```python
from build123d import *

# Parameters (mm, degrees)
SKETCH_1_R               = 16
SKETCH_1_R_2             = 6.65
EXTRUDE_1_DEPTH          = 24
SKETCH_3_R               = 1.5
CUT_EXTRUDE_2_DEPTH      = 33.984845005
PATTERN_CIRCULAR_1_COUNT = 6
EXTRUDE_START            = -24
EXTRUDE_2_DEPTH          = 24
SKETCH_7_R               = 13
CUT_EXTRUDE_3_DEPTH      = 21.8
EXTRUDE_START_2          = 13.8
SKETCH_15_R              = 13
SKETCH_15_R_2            = 12.25
EXTRUDE_4_DEPTH          = 13.8
SKETCH_11_W              = 20
SKETCH_11_H              = 8.5
CUT_EXTRUDE_4_DEPTH      = 10
FILLET_1_R               = 3
SKETCH_12_R              = 1
CUT_EXTRUDE_5_DEPTH      = 44.081318457
HOLE_WIZARD_M3_1_D       = 2.5
CHAMFER_1_SIZE           = 0.5
SKETCH_19_R              = 11
EXTRUDE_8_DEPTH          = 24
SKETCH_20_R              = 11
CUT_EXTRUDE_8_DEPTH      = 47
SKETCH_21_R              = 11
CUT_EXTRUDE_9_DEPTH      = 60
SKETCH_22_R              = 9.5
CUT_EXTRUDE_10_DEPTH     = 60


with BuildPart() as part:
    # 草图1 → 凸台-拉伸1 (new body)
    with BuildSketch(Plane.XY):
        Circle(SKETCH_1_R)
        Circle(SKETCH_1_R_2, mode=Mode.SUBTRACT)
    extrude(amount=EXTRUDE_1_DEPTH)

    # 草图3 → 切除-拉伸2 (cut, through all)
    with BuildSketch(Plane(origin=(0, 0, 0), x_dir=(-1, 0, 0), z_dir=(0, 0, -1))):
        with Locations((0, 9.5)):
            Circle(SKETCH_3_R)
    cut_extrude_2 = extrude(amount=-CUT_EXTRUDE_2_DEPTH, mode=Mode.SUBTRACT)

    # 阵列(圆周)1: 切除-拉伸2 ×6 about axis
    pattern_circular_1_axis = Axis((0, 0, 0), (0, 0, 1))
    for i in range(1, PATTERN_CIRCULAR_1_COUNT):
        add(cut_extrude_2.rotate(pattern_circular_1_axis, i * 360 / PATTERN_CIRCULAR_1_COUNT), mode=Mode.SUBTRACT)

    # 草图4 → 凸台-拉伸2 (add)
    with BuildSketch(Plane.XY.offset(24).offset(EXTRUDE_START)):
        with BuildLine():
            ThreePointArc((16, 0), (11.313708518, -11.31370848), (5.5e-08, -16))
            Line((5.5e-08, -16), (16, -16))
            Line((16, -16), (16, 0))
        make_face()
        with BuildLine():
            ThreePointArc((5.5e-08, -16), (-11.31370848, -11.313708518), (-16, 0))
            Line((-16, 0), (-16, -16))
            Line((-16, -16), (5.5e-08, -16))
        make_face()
        with BuildLine():
            Line((-16, 16), (-16, 0))
            ThreePointArc((-16, 0), (-11.313708518, 11.31370848), (-5.5e-08, 16))
            Line((-5.5e-08, 16), (-16, 16))
        make_face()
        with BuildLine():
            Line((16, 16), (-5.5e-08, 16))
            ThreePointArc((-5.5e-08, 16), (11.31370848, 11.313708518), (16, 0))
            Line((16, 0), (16, 16))
        make_face()
    extrude(amount=EXTRUDE_2_DEPTH)

    # 草图7 → 切除-拉伸3 (cut)
    with BuildSketch(Plane.XY.offset(24)):
        Circle(SKETCH_7_R)
    extrude(amount=-CUT_EXTRUDE_3_DEPTH, mode=Mode.SUBTRACT)

    # 草图15 → 凸台-拉伸4 (add)
    with BuildSketch(Plane.XY.offset(2.2).offset(EXTRUDE_START_2)):
        Circle(SKETCH_15_R)
        Circle(SKETCH_15_R_2, mode=Mode.SUBTRACT)
    extrude(amount=-EXTRUDE_4_DEPTH)

    # 草图11 → 切除-拉伸4 (cut)
    with BuildSketch(Plane(origin=(0, 16, 0), x_dir=(1, 0, 0), z_dir=(0, 1, 0))):
        with Locations((0, -9.75)):
            Rectangle(SKETCH_11_W, SKETCH_11_H)
    extrude(amount=-CUT_EXTRUDE_4_DEPTH, mode=Mode.SUBTRACT)

    # 圆角1
    fillet_1_edges = [part.edges().sort_by_distance(p)[0] for p in [
        (10, 11.537742925, 5.5),
        (10, 11.537742925, 14),
        (-10, 11.537742925, 14),
        (-10, 11.537742925, 5.5),
    ]]
    fillet(fillet_1_edges, radius=FILLET_1_R)

    # 草图12 → 切除-拉伸5 (cut, through all)
    with BuildSketch(Plane(origin=(0, 16, 0), x_dir=(1, 0, 0), z_dir=(0, 1, 0))):
        with Locations(Location((8, -3.5, 0), (0, 0, 180))):
            Circle(SKETCH_12_R)
        with Locations(Location((8, -19.5, 0), (0, 0, 180))):
            Circle(SKETCH_12_R)
        with Locations(Location((-8, -3.5, 0), (0, 0, 180))):
            Circle(SKETCH_12_R)
        with Locations(Location((-8, -19.5, 0), (0, 0, 180))):
            Circle(SKETCH_12_R)
    extrude(amount=-CUT_EXTRUDE_5_DEPTH, mode=Mode.SUBTRACT)

    # M3 螺纹孔1 (through all)
    with Locations(Plane(origin=(0, 16, 0), x_dir=(1, 0, 0), z_dir=(0, 1, 0))):
        with Locations((8, -3.5), (-8, -3.5), (-8, -19.5), (8, -19.5)):
            Hole(HOLE_WIZARD_M3_1_D / 2)

    # 倒角1
    chamfer_1_edges = [part.edges().sort_by_distance(p)[0] for p in [
        (0, -16, 24),
        (16, -16, 12),
        (16, 0, 0),
        (16, 0, 24),
        (0, -16, 0),
        (-16, -16, 12),
        (-16, 0, 24),
        (-16, 0, 0),
        (0, 16, 0),
        (-16, 16, 12),
        (0, 16, 24),
        (16, 16, 12),
    ]]
    chamfer(chamfer_1_edges, length=CHAMFER_1_SIZE)

    # 草图19 → 凸台-拉伸8 (add)
    with BuildSketch(Plane(origin=(0, 0, 0), x_dir=(-1, 0, 0), z_dir=(0, 0, -1))):
        Circle(SKETCH_19_R)
    extrude(amount=-EXTRUDE_8_DEPTH)

    # 草图20 → 切除-拉伸8 (cut)
    with BuildSketch(Plane.XY.offset(5.5)):
        Circle(SKETCH_20_R)
    extrude(amount=CUT_EXTRUDE_8_DEPTH, mode=Mode.SUBTRACT)

    # 草图21 → 切除-拉伸9 (cut)
    with BuildSketch(Plane.XY.offset(2.2)):
        Circle(SKETCH_21_R)
    extrude(amount=CUT_EXTRUDE_9_DEPTH, mode=Mode.SUBTRACT)

    # 草图22 → 切除-拉伸10 (cut)
    with BuildSketch(Plane(origin=(0, 0, 0), x_dir=(-1, 0, 0), z_dir=(0, 0, -1))):
        Circle(SKETCH_22_R)
    extrude(amount=-CUT_EXTRUDE_10_DEPTH, mode=Mode.SUBTRACT)


solid = part.part
```
Source: CAD feature listing. Evaluate the final solid. Frame: model axes, mm. A direction names the side the tool comes from. Round coordinates to 2 decimals unless told otherwise and drop trailing zeros. Order: outer loops, then holes, each group sorted by start corner. A loop starts at its lowest first (then second) coordinate and runs counter-clockwise, first axis right, second up. Notation, with made-up numbers: (4.5, 45) -> (33.5, 45) arc R18 ccw to (33.5, 55) -> close; hole circle Ø7 at (62, 40.5). An arc over 180 degrees is marked (long way). One line per item, written item: value. Start each with the question number.
Q1. Section query B-B (z = 19.5). Return the cut outline in (x, y).
Q2. Section query A-A (y = -13.5). Return the cut outline in (x, z).
Q3. Draft query along Y for faces 1 (the flat face through (-12, 4, 16)), 2 (the cylindrical face through (-9.155, 12.845, 3.979)), 3 (the cylindrical face through (-4.38, -8.43, 1.08)). Return one class per face: pulls with the +Y half, pulls with the -Y half, needs draft (parallel to the pull), parting line crosses it, or undercut.
Q4. Section query D-D (z = 15.5). Return the cut outline in (x, y).
Q5. Pin query (flat end, axial travel): pin 1 (1.5 mm diameter, centred on x = -8, z = 19.5, fed in from -Y); pin 2 (13 mm diameter, centred on x = 1, y = -3.5, fed in from +Z). Return the tip coordinate at first contact, or that it passes through.
Q6. Material intervals for probe 1 along Z at (x, y) = (-8, -11); probe 2 along X at (y, z) = (-11.5, 19.5); probe 3 along X at (y, z) = (13, 10.5), sorted ascending.
Q7. Access query for faces 4 (the flat face through (10, 12, 10)), 5 (the cylindrical face through (-9.19, -12.96, 3.12)), 6 (the cylindrical face through (-10.316, -7.91, 20.056)). Directions: +Z, -Z, +X, -X, +Y, -Y. A direction counts if a zero-diameter tool reaches every point of the face in a straight line with its end or side. Return the directions, or none.
Q8. Section query C-C (y = -6). Return the cut outline in (x, z), plus the area to 3 significant figures.
Findings below:
1. outline: (-16, -15.5) -> (-15.5, -16) -> (-9.25, -16) -> (-9.25, -9.13) arc R13 cw to (-9.25, 9.13) -> (-9.25, 16) -> (-15.5, 16) -> (-16, 15.5) -> close; (-6.75, -16) -> (6.75, -16) -> (6.75, -11.11) arc R13 cw to (-6.75, -11.11) -> close; (-6.75, 11.11) arc R13 cw to (6.75, 11.11) -> (6.75, 16) -> (-6.75, 16) -> close; (9.25, -16) -> (15.5, -16) -> (16, -15.5) -> (16, 15.5) -> (15.5, 16) -> (9.25, 16) -> (9.25, 9.13) arc R13 cw to (9.25, -9.13) -> close
2. outline: (-16, 0.5) -> (-15.5, 0) -> (15.5, 0) -> (16, 0.5) -> (16, 23.5) -> (15.5, 24) -> (-15.5, 24) -> (-16, 23.5) -> close; hole circle Ø2.5 at (-8, 3.5); hole circle Ø2.5 at (-8, 19.5); hole circle Ø2.5 at (8, 3.5); hole circle Ø2.5 at (8, 19.5)
3. face 1: undercut
3. face 2: needs draft
3. face 3: undercut
4. outline: (-16, -15.5) -> (-15.5, -16) -> (15.5, -16) -> (16, -15.5) -> (16, 15.5) -> (15.5, 16) -> (-15.5, 16) -> (-16, 15.5) -> close; hole circle Ø24.5 at (0, 0)
5. pin 1: through
5. pin 2: z = 2.2
6. probe 1: 0 to 2.25, 4.75 to 18.25, 20.75 to 24
6. probe 2: -16 to -9.25, -6.75 to -6.06, 6.06 to 6.75, 9.25 to 16
6. probe 3: -16 to -10, 10 to 16
7. face 4: +Y
7. face 5: +Y, -Y
7. face 6: +Z
8. outline: (-16, 0.5) -> (-15.5, 0) -> (-7.37, 0) -> (-7.37, 2.2) -> (-10.68, 2.2) -> (-10.68, 16) -> (-11.53, 16) -> (-11.53, 24) -> (-15.5, 24) -> (-16, 23.5) -> close; (7.37, 0) -> (15.5, 0) -> (16, 0.5) -> (16, 23.5) -> (15.5, 24) -> (11.53, 24) -> (11.53, 16) -> (10.68, 16) -> (10.68, 2.2) -> (7.37, 2.2) -> close
8. area: 256 mm²
